Design review of the part shown in the three views and the two pictorial views. Dimensions are in mm from the part's minimum x, y and z. Give positions to 0.01 mm unless a question says otherwise; leave off trailing zeros. Write each loop counter-clockwise with the first axis right and the second up, starting at its lowest first coordinate (ties: lowest second). Pieces come first, ordered by that corner, then holes. Notation, with made-up numbers: M 54,34.5 L 69,34.5 A25 ccw 69,47.5 Z; hole C 40.25,29 d6. An arc over 180 degrees is marked long. Write item = value, one per line.
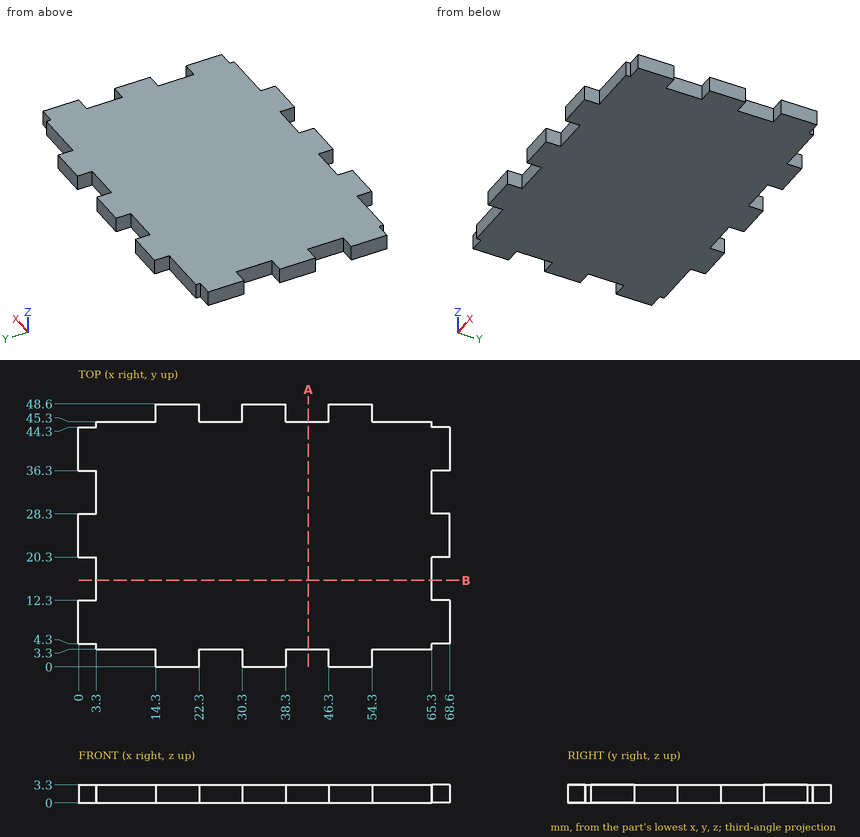
1. Insertion check: P1, Ø1.6, axis at x = 67, z = 1, coming from the -Y side; P2, Ø1.6, axis at x = 58.5, z = 2.5, coming from the +Y side; P3, Ø1.6, axis at x = 58.5, z = 2, coming from the -Y side; P4, Ø5, axis at x = 36, y = 33, coming from the -Z side. Each pin has a flat end and moves straight along its axis. Give the tip position at first contact, or say it passes through.
Responses:
P1 = 4.3
P2 = 45.3
P3 = 3.3
P4 = 0
2. We need section B-B, the plane y = 16. Write out the cut boundary in (x, z), then the cut area to 3 significant figures.
Responses:
outline = M 3.3,0 L 65.3,0 L 65.3,3.3 L 3.3,3.3 Z
area = 205 mm2
3. For line 1 along X through (y, z) = (18.5, 1.6); line 2 along Y through (x, z) = (25, 0.5), list the stretches that pass through material, from the lowest coordinate up. Write a range as from..to.
Responses:
line_1 = 3.3..65.3
line_2 = 3.3..45.3
4. We need section A-A, the plane x = 42.5. Write out the cut boundary in (y, z).
Responses:
outline = M 3.3,0 L 45.3,0 L 45.3,3.3 L 3.3,3.3 Z
